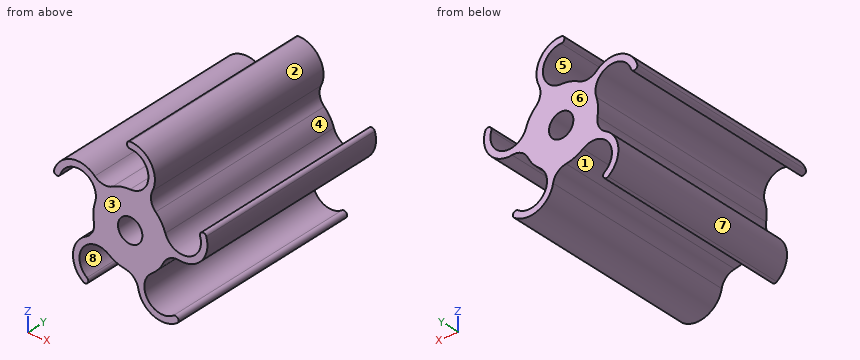
from build123d import *

# Parameters (mm, degrees)
F0_R     = 2
F1_DEPTH = 33


with BuildPart() as f1:
    # F0 (on Front) → F1 (new body)
    with BuildSketch(Plane.XZ):
        with BuildLine():
            ThreePointArc((0, 12.0625), (3, 9.0625), (0, 6.0625))
            ThreePointArc((0, 6.0625), (-1.486924, 5.877326), (-2.883015, 5.333117))
            ThreePointArc((-2.883015, 5.333117), (-4.408233, 5.055069), (-5.804101, 5.729721))
            ThreePointArc((-5.804101, 5.729721), (-9.606608, 6.74108), (-12.482617, 4.055848))
            ThreePointArc((-12.482617, 4.055848), (-12.141533, 3.386434), (-11.472119, 3.727517))
            ThreePointArc((-11.472119, 3.727517), (-7.691899, 5.653636), (-5.76578, 1.873416))
            ThreePointArc((-5.76578, 1.873416), (-6.049154, 0.402045), (-5.962996, -1.093886))
            ThreePointArc((-5.962996, -1.093886), (-6.169875, -2.630377), (-7.242855, -3.749447))
            ThreePointArc((-7.242855, -3.749447), (-9.379753, -7.053318), (-7.714681, -10.618348))
            ThreePointArc((-7.714681, -10.618348), (-6.97263, -10.500819), (-7.09016, -9.758767))
            ThreePointArc((-7.09016, -9.758767), (-7.753855, -5.568361), (-3.563448, -4.904666))
            ThreePointArc((-3.563448, -4.904666), (-2.251659, -5.628849), (-0.802319, -6.009175))
            ThreePointArc((-0.802319, -6.009175), (0.595041, -6.680731), (1.327771, -8.047007))
            ThreePointArc((1.327771, -8.047007), (3.809601, -11.100271), (7.714681, -10.618348))
            ThreePointArc((7.714681, -10.618348), (7.832211, -9.876297), (7.09016, -9.758767))
            ThreePointArc((7.09016, -9.758767), (2.899753, -9.095072), (3.563448, -4.904666))
            ThreePointArc((3.563448, -4.904666), (4.657553, -3.880865), (5.467135, -2.619988))
            ThreePointArc((5.467135, -2.619988), (6.537631, -1.498542), (8.063462, -1.223877))
            ThreePointArc((8.063462, -1.223877), (11.734216, 0.192974), (12.482617, 4.055848))
            ThreePointArc((12.482617, 4.055848), (11.813203, 4.396932), (11.472119, 3.727517))
            ThreePointArc((11.472119, 3.727517), (9.546001, -0.052703), (5.76578, 1.873416))
            ThreePointArc((5.76578, 1.873416), (5.130184, 3.230343), (4.181195, 4.389934))
            ThreePointArc((4.181195, 4.389934), (3.445437, 5.754581), (3.655723, 7.29061))
            ThreePointArc((3.655723, 7.29061), (3.442543, 11.219535), (0, 13.125))
            ThreePointArc((0, 13.125), (-0.53125, 12.59375), (0, 12.0625))
        make_face()
        Circle(F0_R, mode=Mode.SUBTRACT)
    extrude(amount=F1_DEPTH)


solid = f1.part
The listing builds one solid part. Answer for the finished solid, in the listing's coordinates (mm). Face numbers are marked on the shaded views. A direction names the side the tool comes from. Round coordinates to 2 decimals unless told otherwise and drop trailing zeros. Write each loop counter-clockwise with the first axis right and the second up, starting at its lowest first coordinate (ties: lowest second). Pieces come first, ordered by that corner, then holes. Notation, with made-up numbers: M 81,-15.5 L 94,-15.5 A12 cw 94,0.5 Z; hole C 27,60.5 d10. An arc over 180 degrees is marked long. Write each question's results on one line, items separated by ' | '. Start each with the question number.
Item 1: Straight lines are drawn through the part: probe 1 along Z at (x, y) = (0, -8) (1 decimal); probe 2 along X at (y, z) = (-23, 1.25); probe 3 along X at (y, z) = (-24, 4). For each, find the intervals that lie inside material, in ascending order.
Item 2: Given pin 1 Ø12 at (y, z) = (-24.5, -9) entering from +X; pin 2 Ø3 at (x, y) = (9.5, -13.5) entering from +Z; pin 3 Ø3 at (x, z) = (0, 0) entering from +Y; pin 4 Ø1.5 at (y, z) = (-25, 10.5) entering from +X, each flat-ended and moving along its own axis, determine where each tip first touches the part or whether it passes through.
Item 3: Find section A-A on z = -7. Write down the section's boundary in (x, y).
Item 4: Find section C-C on x = -1.5. Write down the section's boundary in (y, z).
Item 5: The mould has two halves that part along X. Classify the marked faces 6, 7 and 8: +X half, -X half, draft (parallel to the pull), parting line (faces both ways), or undercut.
Item 6: Find section D-D on z = 8.25. Write down the section's boundary in (x, y).
Item 7: Which of the six approach directions +Z, -Z, +X, -X, +Y, -Y give full straight-line access (tool end or side, diameter ignored) to the marked faces 1, 2, 3, 4 and 5?
Item 8: Find section B-B on y = -10. Write down the section's boundary in (x, z) (1 decimal).
Answer block:
1) probe 1: z = -6.3 to -2, 2 to 6.1, 12.1 to 13.1 | probe 2: x = -5.93 to -1.56, 1.56 to 6.05, 11.19 to 12.37 | probe 3: x = -12.5 to -11.37, -5.87 to 4.56, 11.46 to 12.5
2) pin 1: stops at x = 7.93 | pin 2: stops at z = 0.98 | pin 3: passes through | pin 4: stops at x = 4
3) outline: M -9.38,-33 L -8.31,-33 L -8.31,0 L -9.38,0 Z; M 0.88,-33 L 2.35,-33 L 2.35,0 L 0.88,0 Z
4) outline: M -33,-5.87 L 0,-5.87 L 0,-1.32 L -33,-1.32 Z; M -33,1.32 L 0,1.32 L 0,5.87 L -33,5.87 Z
5) face 6: draft | face 7: -X half | face 8: undercut
6) outline: M 2.89,-33 L 3.98,-33 L 3.98,0 L 2.89,0 Z
7) face 1: -Z, +Y, -Y | face 2: +X, +Y, -Y | face 3: +Z, -Z, +X, -X, -Y | face 4: +Z, +Y, -Y | face 5: +Y, -Y
8) outline: M -12.5,4.1 A0.5 ccw -11.5,3.7 A3 cw -5.8,1.9 A6.1 ccw -6,-1.1 A2.5 cw -7.2,-3.7 A4.1 ccw -7.7,-10.6 A0.5 ccw -7.1,-9.8 A3 cw -3.6,-4.9 A6.1 ccw -0.8,-6 A2.5 cw 1.3,-8 A4.1 ccw 7.7,-10.6 A0.5 ccw 7.1,-9.8 A3 cw 3.6,-4.9 A6.1 ccw 5.5,-2.6 A2.5 cw 8.1,-1.2 A4.1 ccw 12.5,4.1 A0.5 ccw 11.5,3.7 A3 cw 5.8,1.9 A6.1 ccw 4.2,4.4 A2.5 cw 3.7,7.3 A4.1 ccw 0,13.1 A0.5 ccw 0,12.1 A3 cw 0,6.1 A6.1 ccw -2.9,5.3 A2.5 cw -5.8,5.7 A4.1 ccw Z; hole C 0,0 d4
